The drawing under review shows one solid part. Ordinate dimensions are in mm from its lowest x, y, z. Give positions to 0.01 mm unless a question says otherwise; leave off trailing zeros. Order: outer loops, then holes, each group sorted by start corner. A loop starts at its lowest first (then second) coordinate and runs counter-clockwise, first axis right, second up. Notation, with made-up numbers: (-32.75, 70) -> (20.25, 70) arc R27 cw to (20.25, 107) -> close; hole circle Ø6 at (49, 53). An arc over 180 degrees is marked (long way). Return JSON: item names as keys, results as strings. Group by question number.
1) Add section B-B (y = 87). Give the boundary of the cut face in (x, z).
2) To check wall thickness, follow line 1 along Z through (x, y) = (33.5, 156); line 2 along X through (y, z) = (22, 9.5); line 3 along Y through (x, z) = (10, 32). State the ranges of each line that lie inside material, in increasing order.
3) Insertion check: P1, Ø15.5, axis at y = 27.5, z = 18.5, coming from the +X side; P2, Ø1.9, axis at y = 41.25, z = 34.49, coming from the +X side; P3, Ø17.5, axis at x = 17.5, y = 53.5, coming from the +Z side; P4, Ø1.8, axis at x = 10.5, z = 25, coming from the +Y side. Each pin has a flat end and moves straight along its axis. Give the tip position at first contact, or say it passes through.
4) Add section A-A (z = 29). Give the boundary of the cut face in (x, y), then the cut area to 3 significant figures.
5) The part is to be moulded in two halves that separate along X. For the marked faces 1, 2 and 3, say which applies: released by +X, released by -X, zero draft, split by the parting line, or undercut.
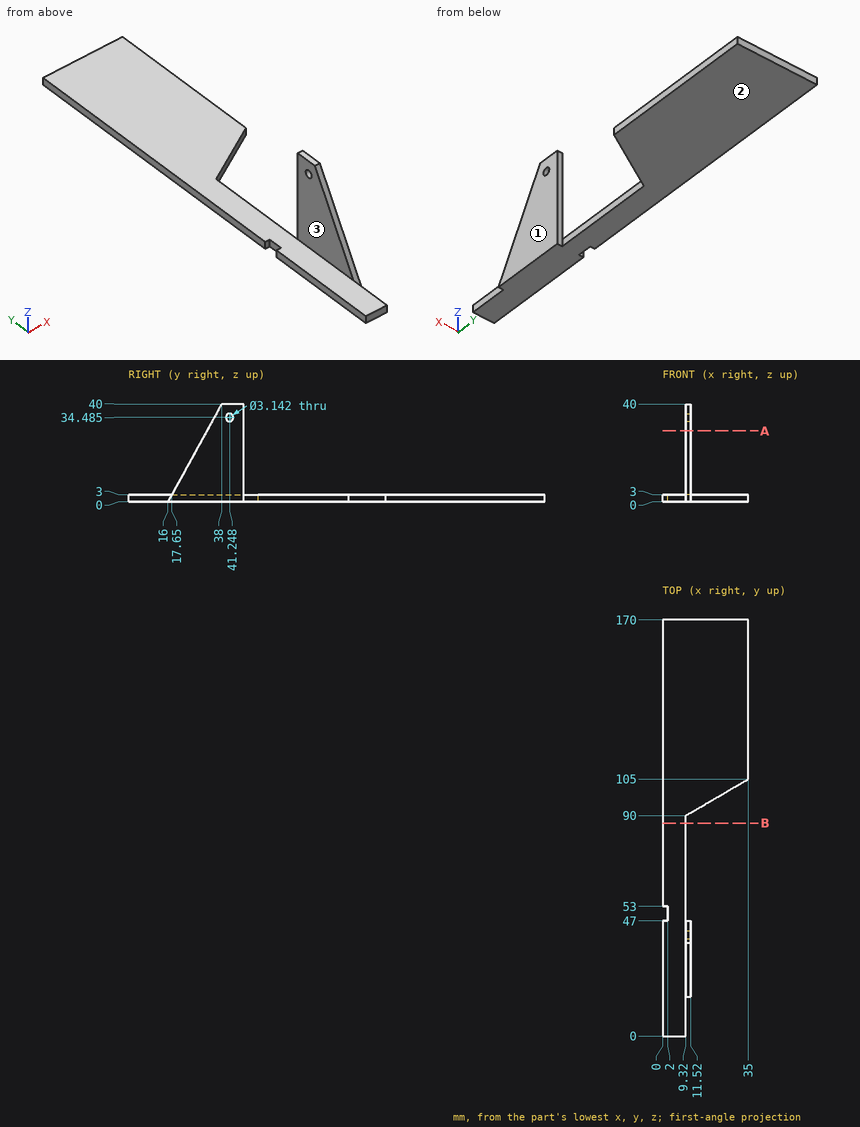
Evaluation:
{
 "1": {"outline": "(0, 0) -> (9.32, 0) -> (9.32, 3) -> (0, 3) -> close"},
 "2": {"line 1": "0 to 3", "line 2": "9.32 to 11.52", "line 3": "33.6 to 47"},
 "3": {"P1": "x = 11.52", "P2": "through", "P3": "z = 3", "P4": "y = 47"},
 "4": {"outline": "(9.32, 31.95) -> (11.52, 31.95) -> (11.52, 47) -> (9.32, 47) -> close", "area": "33.1 mm^2"},
 "5": {"face 1": "released by +X", "face 2": "zero draft", "face 3": "released by -X"}
}
